Geometry: final body of the model. Coordinates: model frame, mm. Face numbers are marked on the shaded views. A direction names the side the tool comes from. Give positions to 0.01 mm unless a question says otherwise; leave off trailing zeros. Order: outer loops, then holes, each group sorted by start corner. A loop starts at its lowest first (then second) coordinate and runs counter-clockwise, first axis right, second up. Notation, with made-up numbers: (-19, -6.75) -> (35, -6.75) arc R16 cw to (35, 4.25) -> close; hole circle Ø3 at (8, 49). An arc over 180 degrees is marked (long way). Write item = value, one per line.
```python
from build123d import *

# Parameters (mm, degrees)
SKETCH_1_R      = 6.75
SKETCH_1_R_2    = 5.25
EXTRUDE_1_DEPTH = 9
SKETCH_2_R      = 0.925
EXTRUDE_2_DEPTH = 9
FILLET_1_R      = 1
EXTRUDE_START   = -1
SKETCH_3_R      = 7.5
SKETCH_3_R_2    = 6.75
EXTRUDE_3_DEPTH = 1
FILLET_2_R      = 1


with BuildPart() as part:
    # 草图1 → 凸台-拉伸1 (new body)
    with BuildSketch(Plane.XY):
        Circle(SKETCH_1_R)
        Circle(SKETCH_1_R_2, mode=Mode.SUBTRACT)
    extrude(amount=EXTRUDE_1_DEPTH)

    # 草图2 → 凸台-拉伸2 (add)
    with BuildSketch(Plane.XY.offset(9)):
        with BuildLine():
            ThreePointArc((0, 2.325), (-1.415370322, 1.844546516), (-2.245777546, 0.60175428))
            Line((-2.245777546, 0.60175428), (-5.780506882, 1.548882151))
            Line((-5.780506882, 1.548882151), (-6.206011413, -0.039122381))
            Line((-6.206011413, -0.039122381), (-2.013509064, -1.1625))
            ThreePointArc((-2.013509064, -1.1625), (-0.88973898, -2.148019913), (0.60175428, -2.245777546))
            Line((0.60175428, -2.245777546), (1.548882151, -5.780506882))
            Line((1.548882151, -5.780506882), (3.136886683, -5.35500235))
            Line((3.136886683, -5.35500235), (2.013509064, -1.1625))
            ThreePointArc((2.013509064, -1.1625), (2.305109303, 0.303473397), (1.644023266, 1.644023266))
            Line((1.644023266, 1.644023266), (4.231624731, 4.231624731))
            Line((4.231624731, 4.231624731), (3.069124731, 5.394124731))
            Line((3.069124731, 5.394124731), (0, 2.325))
        make_face()
        Circle(SKETCH_2_R, mode=Mode.SUBTRACT)
    extrude(amount=-EXTRUDE_2_DEPTH)

    # 圆角1
    fillet_1_edges = [part.edges().sort_by_distance(p)[0] for p in [
        (0.60175428, -2.245777546, 4.5),
        (-2.013509064, -1.1625, 4.5),
        (-5.071110588, 1.358799987, 4.5),
        (-2.245777546, 0.60175428, 4.5),
        (0, 2.325, 4.5),
        (3.712310601, 3.712310601, 4.5),
        (1.644023266, 1.644023266, 4.5),
        (2.013509064, -1.1625, 4.5),
        (1.358799987, -5.071110588, 4.5),
    ]]
    fillet(fillet_1_edges, radius=FILLET_1_R)

    # 草图3 → 凸台-拉伸3 (add)
    with BuildSketch(Plane.XY.offset(9).offset(EXTRUDE_START)):
        Circle(SKETCH_3_R)
        Circle(SKETCH_3_R_2, mode=Mode.SUBTRACT)
    extrude(amount=EXTRUDE_3_DEPTH)

    # 圆角2
    fillet_2_edges = [part.edges().sort_by_distance(p)[0] for p in [
        (-5.241561446, -0.297545971, 4.5),
        (2.363098353, 4.688098353, 4.5),
        (2.878463093, -4.390552382, 4.5),
    ]]
    fillet(fillet_2_edges, radius=FILLET_2_R)


solid = part.part
```
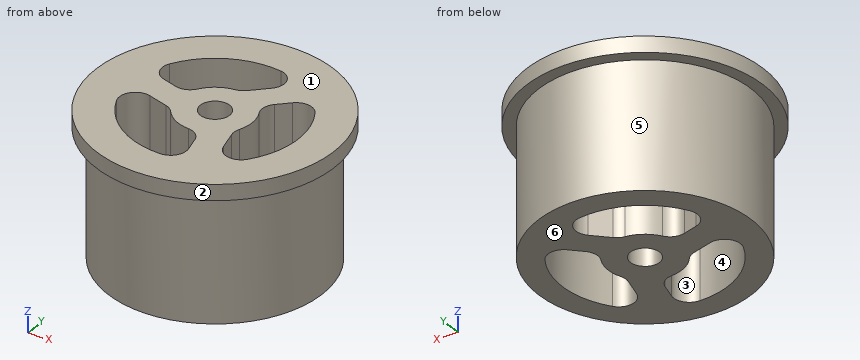
1) Section query B-B (z = 8.25). Output: boundary loops of the cut face in (x, y) (3 decimals).
Check sheet entries:
outline = circle Ø15 at (0, 0); hole (-4.816, -2.091) arc R5.25 ccw to (0.127, -5.248) arc R1 ccw to (1.069, -3.99) -> (0.821, -3.063) arc R1 ccw to (-0.102, -2.323) arc R2.325 cw to (-1.84, -1.421) arc R1 ccw to (-2.373, -1.066) -> (-3.64, -0.727) arc R1 ccw to start; hole (-4.609, 2.514) arc R1 ccw to (-3.99, 1.069) -> (-3.063, 0.821) arc R1 ccw to (-1.961, 1.249) arc R2.325 cw to (-0.31, 2.304) arc R1 ccw to (0.263, 2.588) -> (1.19, 3.515) arc R1 ccw to (0.597, 5.216) arc R5.25 ccw to start; hole circle Ø1.85 at (0, 0); hole (2.062, 1.073) arc R2.325 cw to (2.151, -0.883) arc R1 ccw to (2.11, -1.522) -> (2.449, -2.789) arc R1 ccw to (4.219, -3.125) arc R5.25 ccw to (4.482, 2.735) arc R1 ccw to (2.921, 2.921) -> (2.242, 2.242) arc R1 ccw to start
2) Line query: line 1 (Y direction, x = 0, z = 3.25) (3 decimals); line 2 (X direction, y = -3.25, z = 6); line 3 (X direction, y = 2, z = 2.5). Output: solid intervals per line, ascending. Write a range as from..to.
Check sheet entries:
line_1 = -6.75..-5.25, -2.332..-0.925, 0.925..2.399, 5.25..6.75
line_2 = -5.92..-4.12, 0.87..2.72, 4.11..5.92
line_3 = -6.45..-4.73, -1.19..2.06, 4.85..6.45
3) Reachability of the marked faces 4, 5 and 6 from +Z, -Z, +X, -X, +Y, -Y: full face, straight path, thin tool, end or side. Return the list, or none.
Check sheet entries:
face_4 = +Z, -Z
face_5 = -Z
face_6 = -Z, +X, -X, +Y, -Y
4) Mould query, pull axis Y, two halves, no side actions, for the marked faces 1, 2 and 3. Classes: +Y half, -Y half, draft (parallel to the pull), parting line (faces both ways), or undercut.
Check sheet entries:
face_1 = draft
face_2 = parting line
face_3 = undercut
5) First-contact query: P1, Ø1.5, axis at x = -6, z = 8, coming from the -Y side; P2, Ø4, axis at y = -5, z = 4.5, coming from the -X side; P3, Ø1, axis at y = -3, z = 6, coming from the +X side. Flat tips, straight axial feed; report the tip coordinate or a pass-through.
Check sheet entries:
P1 = -5.36
P2 = -6.05
P3 = 6.27
6) Section query A-A (y = 0). Output: boundary loops of the cut face in (x, z) (3 decimals).
Check sheet entries:
outline = (-7.5, 8) -> (-6.75, 8) -> (-6.75, 0) -> (-0.925, 0) -> (-0.925, 9) -> (-7.5, 9) -> close; (0.925, 0) -> (2.325, 0) -> (2.325, 9) -> (0.925, 9) -> close; (5.25, 0) -> (6.75, 0) -> (6.75, 8) -> (7.5, 8) -> (7.5, 9) -> (5.25, 9) -> close
